Solid Edge part; units mm, degrees
sketch "Sketch1" plane through (0, 0, 0) normal (0, -1, 0) x (1, 0, 0)
  line L0 (2, 16) -> (2, 2)
  line L1 (2, 2) -> (2, 0)
  line L2 (2, 0) -> (0, 0)
  line L3 (-4, 0) -> (0, 0)
  line L4 (-4, -8) -> (-4, 0)
  line L5 (-6, -8) -> (-4, -8)
  line L6 (-6, 2) -> (-6, -8)
  line L7 (0, 2) -> (-6, 2)
  line L8 (0, 2) -> (0, 16)
  line L9 (0, 16) -> (2, 16)
extrude "Protrusion1" add sketch "Sketch1" along normal mid plane 15
sketch "Sketch2" plane through (0, 0, 0) normal (1, 0, 0) x (0, 1, 0)
  circle A0 centre (0, 8.5) radius 3.7
extrude "Cutout1" cut sketch "Sketch2" along normal up to next
fillet "Round_1" radius 5 2 edges at (1, -7.5, 16) (1, 7.5, 16)
Input: part model. Units: mm. Frame: model coordinates. A direction names the side the tool comes from. Coordinates: 2 decimals unless noted, no trailing zeros. Write each loop counter-clockwise with the first axis right and the second up, starting at its lowest first coordinate (ties: lowest second). Pieces come first, ordered by that corner, then holes. Notation, with made-up numbers: M 49.5,-14 L 84.5,-14 A25 cw 84.5,2 Z; hole C 34,82 d10. An arc over 180 degrees is marked long. Answer as a JSON object with one key per item and string values. Group by question number.
(1) Mould query, pull axis Y, two halves, no side actions, for faces 4 (the face through (0.99, -0.48, 4.83)), 5 (the face through (-2, -7.5, 1)), 6 (the face through (-2, 7.5, 1)), 7 (the face through (-1, 0, 0)). Classes: pulls with the +Y half, pulls with the -Y half, needs draft (parallel to the pull), parting line crosses it, or undercut.
(2) Section D-D on z = 11.5. Output: boundary loops of the cut face in (x, y).
(3) Contact query for flat-ended pins moving along their axis: P1, Ø3, axis at x = -1.5, y = 1, coming from the -Z side; P2, Ø1.5, axis at x = 1, z = 13, coming from the -Y side; P3, Ø7, axis at y = 0.5, z = 6.5, coming from the -X side. Output: stop coordinate, or through.
(4) Set-up query: faces 1 (the face through (-4, 0, -4)), 2 (the face through (2, 0.1, 4.6)), 3 (the face through (0, 2, 12)). Return all of +Z, -Z, +X, -X, +Y, -Y with unobstructed straight access to the full face (end or side cutting, diameter ignored); none if empty.
(5) Section B-B on x = 1. Output: boundary loops of the cut face in (y, z), plus the area to 3 significant figures.
(6) Section A-A on z = 8.5. Output: boundary loops of the cut face in (x, y), plus the area to 3 significant figures.
(7) Section C-C on y = 0. Output: boundary loops of the cut face in (x, z).
(8) Ray query, line 1 along Y through (x, z) = (1.1, 8.5); line 2 along Z through (x, y) = (0.9, 0); line 3 along Z through (x, y) = (-5.25, -1.25). Return the intervals inside material, ascending. Write a range as [from, to].
Result set:
{
 "1": {"face 4": "undercut", "face 5": "pulls with the -Y half", "face 6": "pulls with the +Y half", "face 7": "needs draft"},
 "2": {"outline": "M 0,-7.47 L 2,-7.47 L 2,-2.17 L 0,-2.17 Z; M 0,2.17 L 2,2.17 L 2,7.47 L 0,7.47 Z"},
 "3": {"P1": "stops at z = 0", "P2": "stops at y = -7.34", "P3": "stops at x = 0"},
 "4": {"face 1": "-Z, +X, +Y, -Y", "face 2": "+Z, -Z, +X, +Y, -Y", "face 3": "+Z, -X, +Y, -Y"},
 "5": {"outline": "M -7.5,0 L 7.5,0 L 7.5,11 A5 ccw 2.5,16 L -2.5,16 A5 ccw -7.5,11 Z; hole C 0,8.5 d7.4", "area": "186 mm2"},
 "6": {"outline": "M 0,-7.5 L 2,-7.5 L 2,-3.7 L 0,-3.7 Z; M 0,3.7 L 2,3.7 L 2,7.5 L 0,7.5 Z", "area": "15.2 mm2"},
 "7": {"outline": "M -6,-8 L -4,-8 L -4,0 L 2,0 L 2,4.8 L 0,4.8 L 0,2 L -6,2 Z; M 0,12.2 L 2,12.2 L 2,16 L 0,16 Z"},
 "8": {"line 1": "y = [-7.5, -3.7], [3.7, 7.5]", "line 2": "z = [0, 4.8], [12.2, 16]", "line 3": "z = [-8, 2]"}
}
